```python
from build123d import *

# Parameters (mm, degrees)
F0_W         = 44.45
F0_H         = 19.05
F0_R         = 2.38125
F1_DEPTH     = 0.79375
F2_DEPTH     = 4.1402
F3_R         = 5.08
F4_T1_DEPTH  = 40.64
F4_T3_DEPTH  = 15.24
F4_T6_ANGLE  = 90
F4_T8_ANGLE  = 90
F4_T10_ANGLE = 90
F4_T12_ANGLE = 90


# Not quite as in the source:
# - a fillet or chamfer that OpenCascade refuses, or shapes differently, is made with other operations: its cross-section is extruded or revolved along the edge and cut away or added


with BuildPart() as f1:
    # F0 (on Top) → F1 (new body)
    with BuildSketch(Plane.XY):
        with Locations((25.4, 11.0452919405)):
            Rectangle(F0_W, F0_H)
        with Locations((7.14375, 11.8726459702)):
            Circle(F0_R, mode=Mode.SUBTRACT)
    extrude(amount=F1_DEPTH)

    # F0 (on Top) → F2 (join)
    with BuildSketch(Plane.XY):
        Polygon((0, 23.7452919405), (0, 0), (0, -1.6547080595), (50.8, -1.6547080595), (50.8, 23.7452919405), align=None)
        with Locations((25.4, 11.0452919405)):
            Rectangle(F0_W, F0_H, mode=Mode.SUBTRACT)
    extrude(amount=F2_DEPTH)

    # F3
    f3_edges = [f1.edges().sort_by_distance(p)[0] for p in [
        (50.8, -1.654708, 2.0701),
        (0, -1.654708, 2.0701),
        (50.8, 23.745292, 2.0701),
        (0, 23.745292, 2.0701),
    ]]
    fillet(f3_edges, radius=F3_R)

    # F4: fillet of radius 2.54 on 8 edges, made by hand

    # F4_s2 → F4_t1 (cut)
    with BuildSketch(Plane.YZ.offset(5.08)):
        with BuildLine():
            ThreePointArc((-1.6547080595, 1.6002), (-0.9107592837, 3.3962512242), (0.8852919405, 4.1402))
            Line((0.8852919405, 4.1402), (-1.6547080595, 4.1402))
            Line((-1.6547080595, 4.1402), (-1.6547080595, 1.6002))
        make_face()
        with BuildLine():
            ThreePointArc((23.7452919405, 1.6002), (23.0013431647, 3.3962512242), (21.2052919405, 4.1402))
            Line((21.2052919405, 4.1402), (23.7452919405, 4.1402))
            Line((23.7452919405, 4.1402), (23.7452919405, 1.6002))
        make_face()
    extrude(amount=F4_T1_DEPTH, mode=Mode.SUBTRACT)

    # F4_s4 → F4_t3 (cut)
    with BuildSketch(Plane.XZ.offset(-18.6652919405)):
        with BuildLine():
            ThreePointArc((0, 1.6002), (0.7439487758, 3.3962512242), (2.54, 4.1402))
            Line((2.54, 4.1402), (0, 4.1402))
            Line((0, 4.1402), (0, 1.6002))
        make_face()
        with BuildLine():
            ThreePointArc((50.8, 1.6002), (50.0560512242, 3.3962512242), (48.26, 4.1402))
            Line((48.26, 4.1402), (50.8, 4.1402))
            Line((50.8, 4.1402), (50.8, 1.6002))
        make_face()
    extrude(amount=F4_T3_DEPTH, mode=Mode.SUBTRACT)

    # F4_s5 → F4_t6 (revolve, cut)
    with BuildSketch(Plane.XZ.offset(-18.6652919405)):
        with BuildLine():
            ThreePointArc((0, 1.6002), (0.7439487758, 3.3962512242), (2.54, 4.1402))
            Line((2.54, 4.1402), (0, 4.1402))
            Line((0, 4.1402), (0, 1.6002))
        make_face()
    revolve(axis=Axis((5.08, 18.6652919405, 4.1402), (0, 0, -1)), revolution_arc=F4_T6_ANGLE, mode=Mode.SUBTRACT)

    # F4_s7 → F4_t8 (revolve, cut)
    with BuildSketch(Plane.XZ.offset(-3.4252919405)):
        with BuildLine():
            ThreePointArc((0, 1.6002), (0.7439487758, 3.3962512242), (2.54, 4.1402))
            Line((2.54, 4.1402), (0, 4.1402))
            Line((0, 4.1402), (0, 1.6002))
        make_face()
    revolve(axis=Axis((5.08, 3.4252919405, 4.1402), (0, 0, 1)), revolution_arc=F4_T8_ANGLE, mode=Mode.SUBTRACT)

    # F4_s9 → F4_t10 (revolve, cut)
    with BuildSketch(Plane.XZ.offset(-18.6652919405)):
        with BuildLine():
            ThreePointArc((50.8, 1.6002), (50.0560512242, 3.3962512242), (48.26, 4.1402))
            Line((48.26, 4.1402), (50.8, 4.1402))
            Line((50.8, 4.1402), (50.8, 1.6002))
        make_face()
    revolve(axis=Axis((45.72, 18.6652919405, 4.1402), (0, 0, 1)), revolution_arc=F4_T10_ANGLE, mode=Mode.SUBTRACT)

    # F4_s11 → F4_t12 (revolve, cut)
    with BuildSketch(Plane.YZ.offset(45.72)):
        with BuildLine():
            ThreePointArc((-1.6547080595, 1.6002), (-0.9107592837, 3.3962512242), (0.8852919405, 4.1402))
            Line((0.8852919405, 4.1402), (-1.6547080595, 4.1402))
            Line((-1.6547080595, 4.1402), (-1.6547080595, 1.6002))
        make_face()
    revolve(axis=Axis((45.72, 3.4252919405, 4.1402), (0, 0, 1)), revolution_arc=F4_T12_ANGLE, mode=Mode.SUBTRACT)


solid = f1.part
```
Could you check a few things on this model? Use its own coordinates, in mm. A direction names the side the tool comes from. Give positions to 0.01 mm unless a question says otherwise; leave off trailing zeros. Loops run counter-clockwise (first coordinate to the right, second up) from the corner with the lowest first, then second, coordinate; pieces in that order, holes last. Notation, with made-up numbers: (57, 1) -> (109, 1) arc R16 cw to (109, 29) -> close; hole circle Ø4 at (35, 32.5). An arc over 180 degrees is marked (long way). Put each result on its own line as item: value.
(1) Imagine slicing it at B-B on x = 36. Write out the boundary of the cut face in (y, z), plus the area to 3 significant figures.
Computed:
outline: (-1.65, 0) -> (23.75, 0) -> (23.75, 1.6) arc R2.54 ccw to (21.21, 4.14) -> (20.57, 4.14) -> (20.57, 0.79) -> (1.52, 0.79) -> (1.52, 4.14) -> (0.89, 4.14) arc R2.54 ccw to (-1.65, 1.6) -> close
area: 38.6 mm^2
(2) For faces 1 (the face through (50.076, 11.152, 3.376)), 2 (the face through (47.625, 11, 2)), which set-ups out of +Z, -Z, +X, -X, +Y, -Y let a thin tool reach every point of the face, with its end or its side?
Computed:
face 1: +Z, +X, +Y, -Y
face 2: +Z
(3) Imagine slicing it at A-A on y = 7.5. Write out the boundary of the cut face in (x, z) (3 decimals), plus the area to 3 significant figures.
Computed:
outline: (0, 0) -> (50.8, 0) -> (50.8, 1.6) arc R2.54 ccw to (48.26, 4.14) -> (47.625, 4.14) -> (47.625, 0.794) -> (3.175, 0.794) -> (3.175, 4.14) -> (2.54, 4.14) arc R2.54 ccw to (0, 1.6) -> close
area: 58.8 mm^2
(4) Please list where these lines run through material, in increasing order: probe 1 along X at (y, z) = (15.75, 1.2) (3 decimals); probe 2 along X at (y, z) = (14.75, 2.6) (3 decimals); probe 3 along Y at (x, z) = (39, 3.85). Write a range as [from, to].
Computed:
probe 1: [0, 3.175], [47.625, 50.8]
probe 2: [0.205, 3.175], [47.625, 50.595]
probe 3: [-0.29, 1.52], [20.57, 22.38]
(5) I'm going to push flat-ended pins straight in: pin 1 Ø7.5 at (x, y) = (7.14, 11.87) entering from +Z; pin 2 Ø1 at (x, z) = (15.5, 3) entering from -Y. Where does each tip first touch, or does it pass through?
Computed:
pin 1: z = 0.79
pin 2: y = -1.49
(6) Thinking about a two-plate mould opening in X: for faces 3 (the face through (3.175, 11, 2)), 4 (the face through (1.45, 22.22, 0.81)), 5 (the face through (25, 11, 0)), which applies, pulls with the +X half, pulls with the -X half, needs draft (parallel to the pull), parting line crosses it, or undercut?
Computed:
face 3: undercut
face 4: pulls with the -X half
face 5: needs draft
